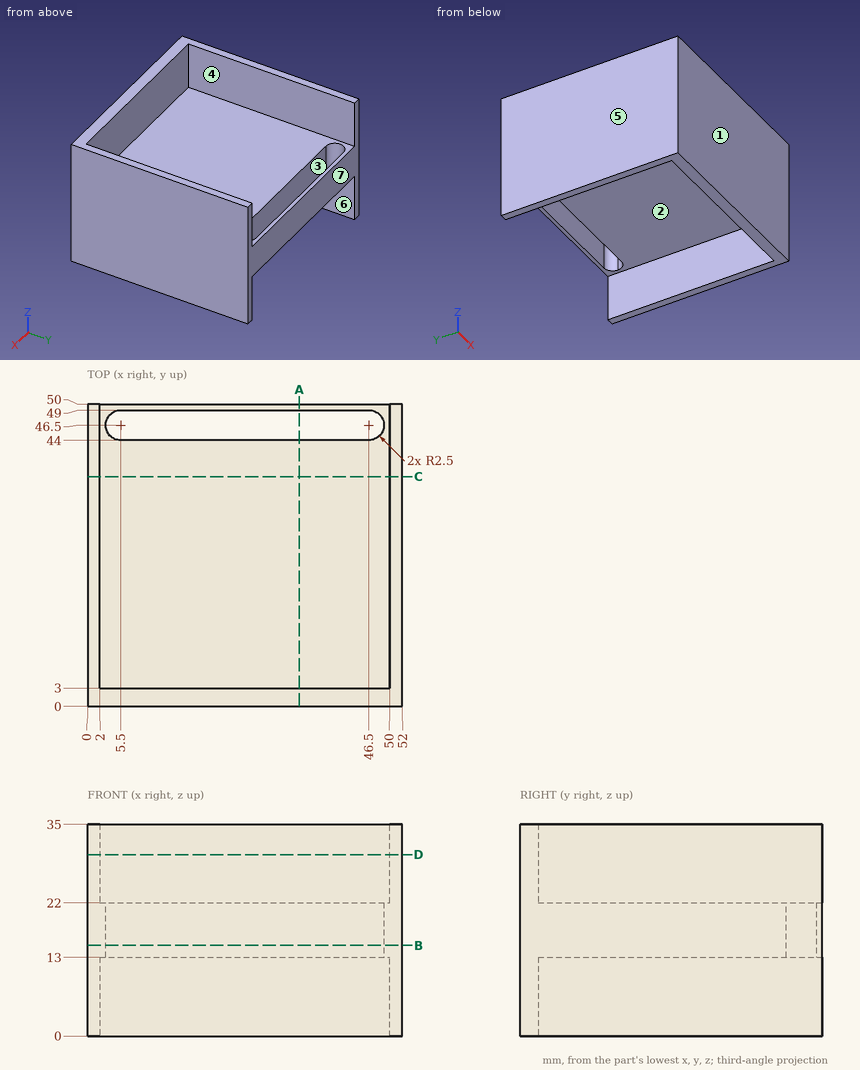
The drawing under review shows one solid part. Ordinate dimensions are in mm from its lowest x, y, z. A direction names the side the tool comes from. Round coordinates to 2 decimals unless told otherwise and drop trailing zeros. Write each loop counter-clockwise with the first axis right and the second up, starting at its lowest first coordinate (ties: lowest second). Pieces come first, ordered by that corner, then holes. Notation, with made-up numbers: (-38, 41.5) - (14, 41.5) arc R31 cw to (14, 72.5) - close; hole circle Ø2 at (35, -17). An arc over 180 degrees is marked (long way). Use one line per item in the form item = value.
Q1. Consider section D-D (z = 30). State the section outline as (x, y) points.
Answer key:
outline = (0, 0) - (52, 0) - (52, 50) - (50, 50) - (50, 3) - (2, 3) - (2, 50) - (0, 50) - close
Q2. Consider section A-A (x = 35). State the section outline as (y, z) points, and give its area (3 significant figures).
Answer key:
outline = (0, 0) - (3, 0) - (3, 13) - (44, 13) - (44, 22) - (3, 22) - (3, 35) - (0, 35) - close; (49, 13) - (50, 13) - (50, 22) - (49, 22) - close
area = 483 mm2
Q3. Consider section B-B (z = 15). State the section outline as (x, y) points, and give its area (3 significant figures).
Answer key:
outline = (0, 0) - (52, 0) - (52, 50) - (0, 50) - close; hole (5.5, 44) - (46.5, 44) arc R2.5 ccw to (46.5, 49) - (5.5, 49) arc R2.5 ccw to start
area = 2,380 mm2
Q4. Tool access review of the marked faces 1, 2, 3 and 4: name each direction out of +Z, -Z, +X, -X, +Y, -Y from which nothing blocks a thin tool from reaching the whole face with its end or side.
Answer key:
face_1 = +Z, -Z, +X, -X, -Y
face_2 = -Z, +Y
face_3 = +Z, -Z
face_4 = +Z, +Y
Q5. For line 1 (Y direction, x = 18, z = 16); line 2 (X direction, y = 26.5, z = 24.5); line 3 (Z direction, x = 28.5, y = 28.5), list the stretches that pass through material, from the lowest coordinate up. Write a range as [from, to].
Answer key:
line_1 = [0, 44], [49, 50]
line_2 = [0, 2], [50, 52]
line_3 = [13, 22]
Q6. Insertion check: pin 1 Ø4 at (x, z) = (22.5, 8.5) entering from +Y; pin 2 Ø23.5 at (x, y) = (14, 16.5) entering from -Z. Each pin has a flat end and moves straight along its axis. Give the tip position at first contact, or say it passes through.
Answer key:
pin_1 = 3
pin_2 = 13
Q7. Draft analysis for pull direction X (two halves, no side actions). For the marked faces 5, 6 and 7, state which applies: +X half, -X half, draft (parallel to the pull), parting line (faces both ways), or undercut.
Answer key:
face_5 = -X half
face_6 = undercut
face_7 = draft
Q8. Consider section C-C (y = 38). State the section outline as (x, z) points, and give its area (3 significant figures).
Answer key:
outline = (0, 0) - (2, 0) - (2, 13) - (50, 13) - (50, 0) - (52, 0) - (52, 35) - (50, 35) - (50, 22) - (2, 22) - (2, 35) - (0, 35) - close
area = 572 mm2
